Check sheet for the modelled part. Datum: model origin and axes. Units: mm. Round coordinates to 2 decimals unless told otherwise and drop trailing zeros. Order: outer loops, then holes, each group sorted by start corner. A loop starts at its lowest first (then second) coordinate and runs counter-clockwise, first axis right, second up.
Q1. Scan lines: probe 1 along X at (y, z) = (-6, 0.05); probe 2 along Y at (x, z) = (25, 0.05); probe 3 along Y at (x, z) = (6.5, 0.05). Record each from-to range of solid material in increasing order.
Q2. Cross-section at B-B on z = 0.05. Record the cut outline in (x, y).
Q3. Cross-section at D-D on y = -3.5. Record the cut outline in (x, z), then the cut area to 3 significant figures.
Q4. Cross-section at C-C on x = 11. Record the cut outline in (y, z).
Q5. Cross-section at A-A on y = -6.5. Record the cut outline in (x, z).
from build123d import *

# Parameters (mm, degrees)
SALIENTE_EXTRUIR1_DEPTH = 0.1


with BuildPart() as part:
    # Model → Saliente-Extruir1 (new body)
    with BuildSketch(Plane.XY):
        with BuildLine():
            Line((33.228973848, 0.17393572), (16.510690428, 0.452082872))
            Line((16.510690428, 0.452082872), (4.649558375, -7.011379622))
            ThreePointArc((4.649558375, -7.011379622), (4.19427636, -8.013126504), (4.9350707, -8.826761725))
            Line((4.9350707, -8.826761725), (9.27203732, -8.826761725))
            Line((9.27203732, -8.826761725), (24.522151852, -8.826761725))
            Line((24.522151852, -8.826761725), (24.522151852, -4.826761725))
            Line((24.522151852, -4.826761725), (27.772151852, -4.826761725))
            Line((27.772151852, -4.826761725), (27.772151852, -8.826761725))
            ThreePointArc((27.772151852, -8.826761725), (29.852156514, -8.399354323), (31.383104023, -6.927859775))
            Line((31.383104023, -6.927859775), (33.228973848, 0.17393572))
        make_face()
    extrude(amount=SALIENTE_EXTRUIR1_DEPTH)


solid = part.part
Results found:
1. probe 1: x = 6.26 to 24.52, 27.77 to 31.62
1. probe 2: y = -4.83 to 0.31
1. probe 3: y = -8.83 to -5.85
2. outline: (4.65, -7.01) arc R1 ccw to (4.94, -8.83) - (24.52, -8.83) - (24.52, -4.83) - (27.77, -4.83) - (27.77, -8.83) arc R3.82 ccw to (31.38, -6.93) - (33.23, 0.17) - (16.51, 0.45) - close
3. outline: (10.23, 0) - (32.27, 0) - (32.27, 0.1) - (10.23, 0.1) - close
3. area: 2.20 mm2
4. outline: (-8.83, 0) - (-3.02, 0) - (-3.02, 0.1) - (-8.83, 0.1) - close
5. outline: (5.46, 0) - (24.52, 0) - (24.52, 0.1) - (5.46, 0.1) - close; (27.77, 0) - (31.49, 0) - (31.49, 0.1) - (27.77, 0.1) - close
